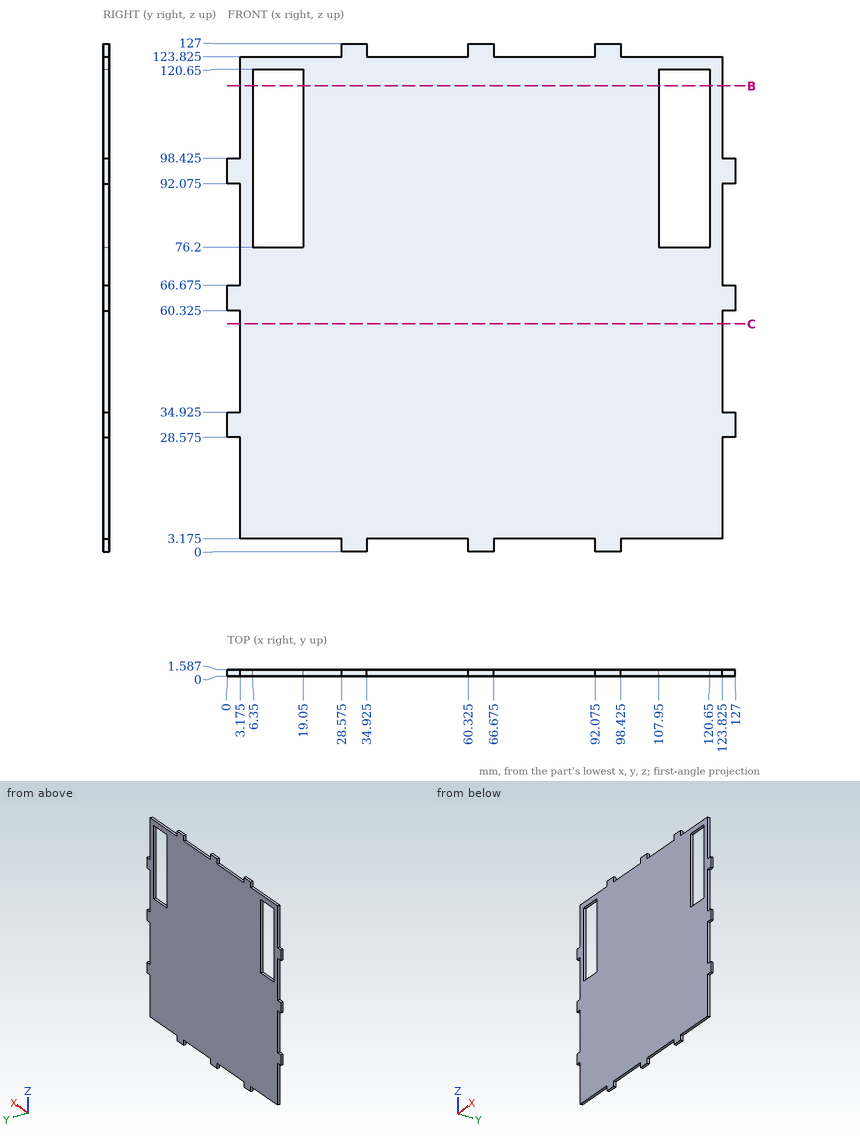
Input: dimensioned drawing with shaded views. Units: mm. Origin: part minimum x, y, z. Round coordinates to 2 decimals unless told otherwise and drop trailing zeros. Order: outer loops, then holes, each group sorted by start corner. A loop starts at its lowest first (then second) coordinate and runs counter-clockwise, first axis right, second up. Notation, with made-up numbers: (-13, -17) - (18, -17) arc R26 ccw to (18, -1) - close; hole circle Ø1 at (-22.5, -32.5). An arc over 180 degrees is marked (long way). Write item = value, one per line. Start each with the question number.
Q1. Pin query (flat end, axial travel): pin 1 (0.8 mm diameter, centred on x = 125, y = 1, fed in from +Z) (1 decimal); pin 2 (0.5 mm diameter, centred on x = 83, y = 1, fed in from -Z) (1 decimal); pin 3 (0.5 mm diameter, centred on y = 1, z = 1, fed in from +X) (1 decimal). Return the tip coordinate at first contact, or that it passes through.
Q2. Cut plane C-C on z = 57. Return the cut outline in (x, y) (1 decimal).
Q3. Cut plane B-B on z = 116.5. Give the number of separate pieces and of enclosed holes in the cut face, and give its area (3 significant figures).
Q4. Ray query, line 1 (X direction, y = 0.1, z = 94.5); line 2 (Z direction, x = 41.5, y = 1.05) (1 decimal). Return the intervals inside material, ascending. Write a range as from..to.
Outcome:
q1.pin_1 = 98.4
q1.pin_2 = 3.2
q1.pin_3 = 98.4
q2.outline = (3.2, 0) - (123.8, 0) - (123.8, 1.6) - (3.2, 1.6) - close
q3.separate_pieces = 3
q3.enclosed_holes = 0
q3.area = 151 mm^2
q4.line_1 = 0..6.35, 19.05..107.95, 120.65..127
q4.line_2 = 3.2..123.8
